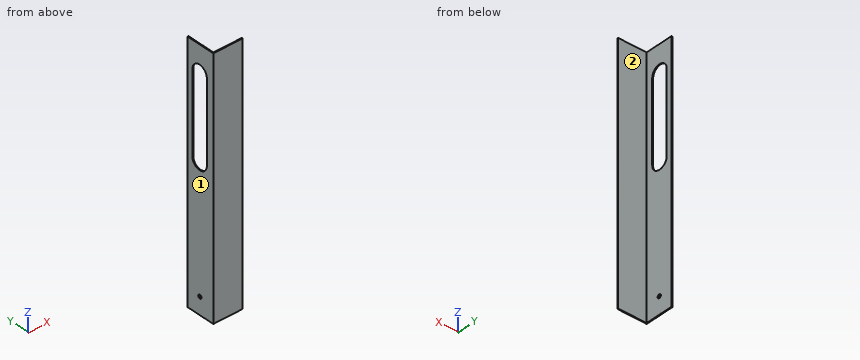
```python
from build123d import *

# Parameters (mm, degrees)
BOSS_EXTRUDE2_DEPTH = 431.8
SKETCH8_R           = 3.175
CUT_EXTRUDE6_DEPTH  = 2.54


with BuildPart() as part:
    # Sketch3 → Boss-Extrude2 (new body)
    with BuildSketch(Plane.XY):
        Polygon((49.2125, 1.5875), (49.2125, 50.8), (50.8, 50.8), (50.8, 1.524), (100.0125, 1.524), (100.0125, 0), (49.2125, 0), align=None)
    extrude(amount=BOSS_EXTRUDE2_DEPTH)

    # Sketch8 → Cut-Extrude6 (cut)
    with BuildSketch(Plane(origin=(50.8, 0, 0), x_dir=(0, 0, -1), z_dir=(1, 0, 0))):
        with Locations((-29.464, 26.416)):
            Circle(SKETCH8_R)
        with BuildLine():
            Line((-245.364, 12.7), (-385.318, 12.7))
            ThreePointArc((-385.318, 12.7), (-399.542, 26.924), (-385.318, 41.148))
            Line((-385.318, 41.148), (-245.364, 41.148))
            ThreePointArc((-245.364, 41.148), (-231.14, 26.924), (-245.364, 12.7))
        make_face()
    extrude(amount=-CUT_EXTRUDE6_DEPTH, mode=Mode.SUBTRACT)


solid = part.part
```
The listing builds one solid part. Answer for the finished solid, in the listing's coordinates (mm). Face numbers are marked on the shaded views. A direction names the side the tool comes from. Round coordinates to 2 decimals unless told otherwise and drop trailing zeros. Loops run counter-clockwise (first coordinate to the right, second up) from the corner with the lowest first, then second, coordinate; pieces in that order, holes last. Notation, with made-up numbers: (-32.75, -20.75) - (18.25, -20.75) arc R12 ccw to (18.25, -11.75) - close; hole circle Ø11 at (4.25, 42.5). An arc over 180 degrees is marked (long way). Use one line per item in the form item = value. Start each with the question number.
1. The part is cut by section A-A on z = 270.5. Determine the outline of the cut face in (x, y), then the cut area to 3 significant figures.
2. Consider line 1 (Y direction, x = 76, z = 138.5); line 2 (X direction, y = 14, z = 157). Determine where each line is inside the solid, lowest interval first. Write a range as [from, to].
3. A tool of negligible diameter and unlimited length cuts with its end or side. For the marked faces 1 and 2, from which of +Z, -Z, +X, -X, +Y, -Y can it reach the whole face along a straight path? Write none if from no direction.
4. The part is cut by section D-D on z = 189. Determine the outline of the cut face in (x, y).
5. The part is cut by section C-C on x = 61.5. Determine the outline of the cut face in (y, z), then the cut area to 3 significant figures.
6. Given pin 1 Ø24.5 at (x, z) = (75, 155.5) entering from +Y; pin 2 Ø1 at (y, z) = (34, 214.5) entering from +X, each flat-ended and moving along its own axis, determine where each tip first touches the part or whether it passes through.
7. The part is cut by section B-B on y = 17. Determine the outline of the cut face in (x, z).
Geometry check:
q1.outline = (49.21, 0) - (100.01, 0) - (100.01, 1.52) - (50.8, 1.52) - (50.8, 12.7) - (49.21, 12.7) - close; (49.21, 41.15) - (50.8, 41.15) - (50.8, 50.8) - (49.21, 50.8) - close
q1.area = 110 mm^2
q2.line_1 = [0, 1.52]
q2.line_2 = [49.21, 50.8]
q3.face_1 = +Z, -Z, -X, +Y, -Y
q3.face_2 = +Z, -Z, +X, +Y
q4.outline = (49.21, 0) - (100.01, 0) - (100.01, 1.52) - (50.8, 1.52) - (50.8, 50.8) - (49.21, 50.8) - close
q5.outline = (0, 0) - (1.52, 0) - (1.52, 431.8) - (0, 431.8) - close
q5.area = 658 mm^2
q6.pin_1 = 1.52
q6.pin_2 = 50.8
q7.outline = (49.21, 0) - (50.8, 0) - (50.8, 235.17) - (49.21, 235.17) - close; (49.21, 395.51) - (50.8, 395.51) - (50.8, 431.8) - (49.21, 431.8) - close
